Here's the drawing with two shaded views (mm, measured from the low corner). I have some questions. A direction names the side the tool comes from. Round coordinates to 2 decimals unless told otherwise and drop trailing zeros. Loops run counter-clockwise (first coordinate to the right, second up) from the corner with the lowest first, then second, coordinate; pieces in that order, holes last. Notation, with made-up numbers: (62.25, -31) - (113.25, -31) arc R31 ccw to (113.25, 2) - close; hole circle Ø11 at (23.5, 76). An arc over 180 degrees is marked (long way). Answer as CSV lines item,"result".
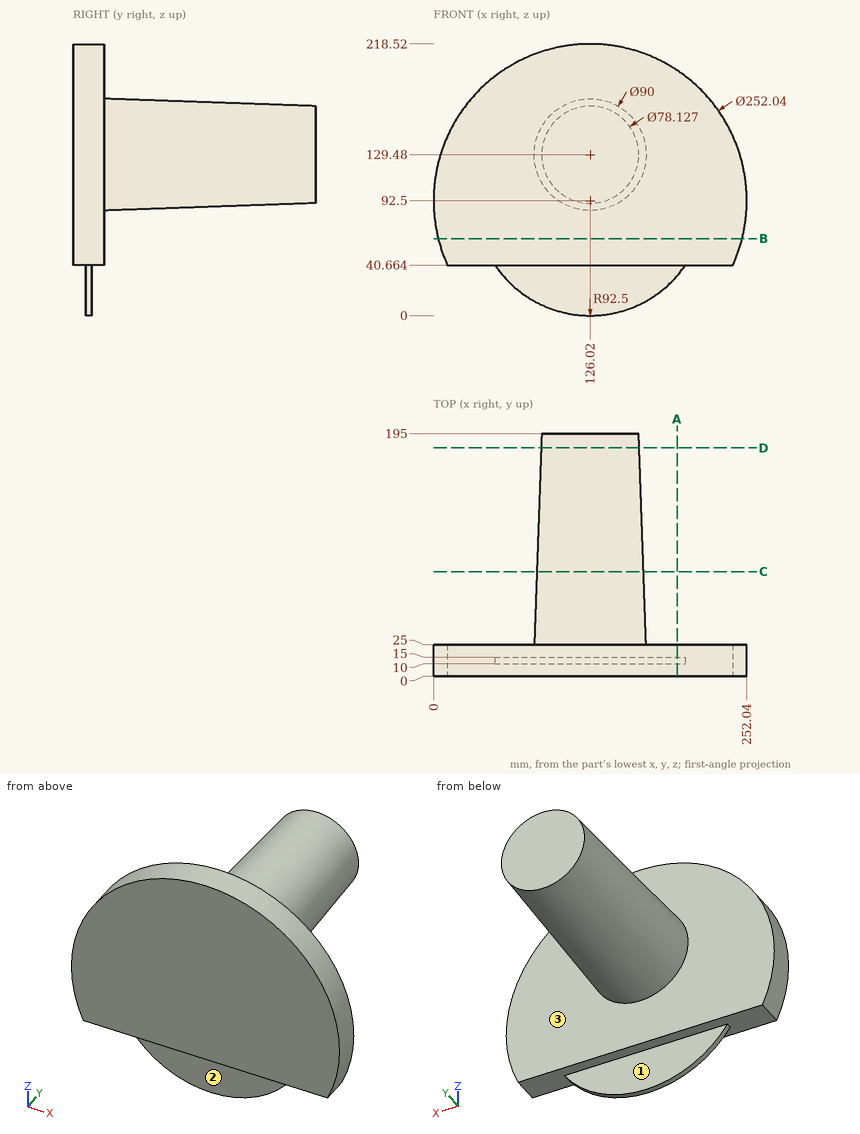
Q1. Imagine slicing it at D-D (y = 183.5). Write out the boundary of the cut face in (x, z) (1 decimal).
Checks:
outline,"circle Ø78.9 at (126, 129.5)"
Q2. Imagine slicing it at B-B (z = 62). Write out the boundary of the cut face in (x, y).
Checks:
outline,"(3.75, 0) - (248.29, 0) - (248.29, 25) - (3.75, 25) - close"
Q3. On a 3-axis mill with a long thin cutter (end or side, diameter ignored), from which of +Z, -Z, +X, -X, +Y, -Y can I reach the whole of each face in a straight line? I mean the marked faces 1, 2 and 3. Say none if no direction works.
Checks:
face 1,"-Z, +X, -X, +Y"
face 2,"-Z, +X, -X, -Y"
face 3,"+Y"
Q4. If I drill on line 1 along Y through (x, z) = (158, 42); line 2 along X through (y, z) = (55, 90) (1 decimal); line 3 along X through (y, z) = (55, 102), over which ranges is the centre line in solid material (lowest first)? Write a range as [from, to].
Checks:
line 1,"[0, 25]"
line 2,"[106.7, 145.3]"
line 3,"[91.72, 160.32]"
Q5. I'm going to push flat-ended pins straight in: pin 1 Ø12 at (x, z) = (149.5, 10.5) entering from -Y; pin 2 Ø4 at (y, z) = (43, 157.5) entering from -X (1 decimal); pin 3 Ø12 at (x, z) = (116.5, 13.5) entering from +Y; pin 4 Ø6 at (x, z) = (98, 158.5) entering from -Y. Where does each tip first touch, or does it pass through?
Checks:
pin 1,"y = 10"
pin 2,"x = 90.1"
pin 3,"y = 15"
pin 4,"y = 0"
Q6. Imagine slicing it at A-A (x = 196). Write out the boundary of the cut face in (y, z).
Checks:
outline,"(0, 40.66) - (10, 40.66) - (10, 32.01) - (15, 32.01) - (15, 40.66) - (25, 40.66) - (25, 197.3) - (0, 197.3) - close"
Q7. Imagine slicing it at C-C (y = 84). Write out the boundary of the cut face in (x, z).
Checks:
outline,"circle Ø85.88 at (126.02, 129.48)"
